```python
from build123d import *

# Parameters (mm, degrees)
BOSS_EXTRUDE1_DEPTH  = 10
FILLET1_R            = 5
SKETCH6_R            = 4.65
BOSS_EXTRUDE2_DEPTH  = 5
SKETCH7_R            = 5
BOSS_EXTRUDE3_DEPTH  = 2
FILLET2_R            = 1
FILLET2_OF_MIRROR1_R = 1
BOSS_EXTRUDE4_START  = -10
BOSS_EXTRUDE4_DEPTH  = 10
SKETCH9_R            = 4.175
CUT_EXTRUDE1_DEPTH   = 5
SKETCH10_R           = 1.175
CUT_EXTRUDE2_DEPTH   = 71.738227722
SKETCH12_W           = 1
SKETCH12_H           = 12
CUT_EXTRUDE3_DEPTH   = 7
CUT_EXTRUDE3_DRAFT   = -2
SKETCH13_W           = 1
SKETCH13_H           = 12
CUT_EXTRUDE4_DEPTH   = 7
CUT_EXTRUDE4_DRAFT   = -2


with BuildPart() as part:
    # Sketch3 → Boss-Extrude1 (new body)
    with BuildSketch(Plane(origin=(0, 0, 0), x_dir=(0, 0, -1), z_dir=(1, 0, 0))):
        with BuildLine():
            Line((-37, -7), (-37, 12.5))
            ThreePointArc((-37, 12.5), (-27.627416998, 35.127416998), (-5, 44.5))
            Line((-5, 44.5), (5, 44.5))
            ThreePointArc((5, 44.5), (27.627416998, 35.127416998), (37, 12.5))
            Line((37, 12.5), (37, -7))
            Line((37, -7), (40, -7))
            Line((40, -7), (40, 12.5))
            ThreePointArc((40, 12.5), (29.748737342, 37.248737342), (5, 47.5))
            Line((5, 47.5), (-5, 47.5))
            ThreePointArc((-5, 47.5), (-29.748737342, 37.248737342), (-40, 12.5))
            Line((-40, 12.5), (-40, -7))
            Line((-40, -7), (-37, -7))
        make_face()
    extrude(amount=BOSS_EXTRUDE1_DEPTH)

    # Fillet1
    fillet1_edges = [part.edges().sort_by_distance(p)[0] for p in [
        (10, -7, -38.5),
        (0, -7, -38.5),
        (0, -7, 38.5),
        (10, -7, 38.5),
    ]]
    fillet(fillet1_edges, radius=FILLET1_R - 0.0001)  # a hair under: the kernel refuses the full size

    # Sketch6 → Boss-Extrude2 (add)
    with BuildSketch(Plane(origin=(0, 0, 37), x_dir=(-1, 0, 0), z_dir=(0, 0, -1))):
        with Locations(Location((-5, 0, 0), (0, 0, 270))):
            Circle(SKETCH6_R)
    boss_extrude2 = extrude(amount=BOSS_EXTRUDE2_DEPTH)

    # Sketch7 → Boss-Extrude3 (add)
    with BuildSketch(Plane(origin=(0, 0, 32), x_dir=(-1, 0, 0), z_dir=(0, 0, -1))):
        with Locations(Location((-5, 0, 0), (0, 0, 90))):
            Circle(SKETCH7_R)
    boss_extrude3 = extrude(amount=BOSS_EXTRUDE3_DEPTH)

    # Fillet2
    fillet2_edges = [part.edges().sort_by_distance(p)[0] for p in [
        (5, -5, 30),
    ]]
    fillet(fillet2_edges, radius=FILLET2_R)

    # Mirror1: Boss-Extrude2, Boss-Extrude3 across plane
    add(boss_extrude2.mirror(Plane.XY))
    add(boss_extrude3.mirror(Plane.XY))

    # Fillet2 of Mirror1
    fillet2_of_mirror1_edges = [part.edges().sort_by_distance(p)[0] for p in [
        (5, -5, -30),
    ]]
    fillet(fillet2_of_mirror1_edges, radius=FILLET2_OF_MIRROR1_R)

    # Sketch8 → Boss-Extrude4 (add)
    with BuildSketch(Plane(origin=(10, 0, 0), x_dir=(0, 0, -1), z_dir=(1, 0, 0)).offset(BOSS_EXTRUDE4_START)):
        with BuildLine():
            Line((8.815238473, 55.479534195), (-8.815238473, 55.479534195))
            add(Edge.make_bspline(
                [(-16.460806571, 45.570378177), (-9.68931269, 49.59059719), (-8.815238473, 55.479534195)],
                knots=[0, 0, 0, 1, 1, 1], degree=2))
            ThreePointArc((-16.460806571, 45.570378177), (-10.811056867, 47.014223417), (-5, 47.5))
            Line((-5, 47.5), (5, 47.5))
            ThreePointArc((5, 47.5), (10.811056867, 47.014223417), (16.460806571, 45.570378177))
            add(Edge.make_bspline(
                [(16.460806571, 45.570378177), (9.68931269, 49.59059719), (8.815238473, 55.479534195)],
                knots=[0, 0, 0, 1, 1, 1], degree=2))
        make_face()
    extrude(amount=BOSS_EXTRUDE4_DEPTH)

    # Sketch9 → Cut-Extrude1 (cut)
    with BuildSketch(Plane(origin=(0, 55.479534195, 0), x_dir=(1, 0, 0), z_dir=(0, 1, 0))):
        with Locations(Location((5, 0, 0), (0, 0, 270))):
            Circle(SKETCH9_R)
    extrude(amount=-CUT_EXTRUDE1_DEPTH, mode=Mode.SUBTRACT)

    # Sketch10 → Cut-Extrude2 (cut, through all)
    with BuildSketch(Plane(origin=(0, 50.479534195, 0), x_dir=(1, 0, 0), z_dir=(0, 1, 0))):
        with Locations(Location((5, 0, 0), (0, 0, 270))):
            Circle(SKETCH10_R)
    extrude(amount=-CUT_EXTRUDE2_DEPTH, mode=Mode.SUBTRACT)


with BuildPart() as cut_extrude3_tool:
    # Sketch12 → Cut-Extrude3 (with draft: the straight prism first)
    with BuildSketch(Plane(origin=(0, 0, 30), x_dir=(-1, 0, 0), z_dir=(0, 0, -1))):
        with Locations((-5, 0)):
            Rectangle(SKETCH12_W, SKETCH12_H)
    extrude(amount=-CUT_EXTRUDE3_DEPTH)
    # Cut-Extrude3: the draft: its side faces are tilted about the plane it starts from
    cut_extrude3_sides = [cut_extrude3_tool.faces().sort_by_distance(p)[0] for p in [
        (4.5, 0, 33.5),
        (5, 6, 33.5),
        (5.5, 0, 33.5),
        (5, -6, 33.5),
    ]]
    draft(cut_extrude3_sides, Plane(origin=(0, 0, 30), x_dir=(-1, 0, 0), z_dir=(0, 0, -1)), CUT_EXTRUDE3_DRAFT)


with BuildPart() as part_1:
    add(part.part)

    # Cut-Extrude3: cut by cut_extrude3_tool
    add(cut_extrude3_tool.part, mode=Mode.SUBTRACT)


with BuildPart() as cut_extrude4_tool:
    # Sketch13 → Cut-Extrude4 (with draft: the straight prism first)
    with BuildSketch(Plane.XY.offset(-30)):
        with Locations((5, 0)):
            Rectangle(SKETCH13_W, SKETCH13_H)
    extrude(amount=-CUT_EXTRUDE4_DEPTH)
    # Cut-Extrude4: the draft: its side faces are tilted about the plane it starts from
    cut_extrude4_sides = [cut_extrude4_tool.faces().sort_by_distance(p)[0] for p in [
        (5, -6, -33.5),
        (5.5, 0, -33.5),
        (5, 6, -33.5),
        (4.5, 0, -33.5),
    ]]
    draft(cut_extrude4_sides, Plane.XY.offset(-30), CUT_EXTRUDE4_DRAFT)


with BuildPart() as part_2:
    add(part_1.part)

    # Cut-Extrude4: cut by cut_extrude4_tool
    add(cut_extrude4_tool.part, mode=Mode.SUBTRACT)


solid = part_2.part
```
CAD build for the part. Positions are in the model's coordinates, mm. A direction names the side the tool comes from. Give positions to 0.01 mm unless a question says otherwise; leave off trailing zeros. Order: outer loops, then holes, each group sorted by start corner. A loop starts at its lowest first (then second) coordinate and runs counter-clockwise, first axis right, second up.
(1) Drill centre lines: L1, parallel to X at y = 48.05, z = 0 (3 decimals); L2, parallel to Z at x = 7, y = 10; L3, parallel to Z at x = 6.75, y = -1. Where is each one in solid material? Low to high.
(2) Saw through at D-D, the plane y = 13.5. Give the cut face in (x, z).
(3) Saw through at B-B, the plane y = 33. Give the cut face in (x, z).
(4) Tool access for faces 1 (the cylindrical face through (0.924, 53.015, -0.905)), 2 (the flat face through (7, 0, -30)), 3 (the cylindrical face through (0.35, -0.1, -34.53)), 4 (the flat face through (9.8, 0, -32)): list every direction of +Z, -Z, +X, -X, +Y, -Y with a clear straight run to the whole face (end or side of a thin tool).
(5) Flat gauge pins, fed straight in: pin 1 (6 mm diameter, centred on x = 8.5, z = -23.5, fed in from -Y); pin 2 (4 mm diameter, centred on x = 7, z = 28.5, fed in from -Y); pin 3 (1.5 mm diameter, centred on x = 6.5, z = 20.5, fed in from +Y). Where does each tip first touch, or does it go through?
(6) Saw through at C-C, the plane z = -34. Give the cut face in (x, y), then the cut area to 3 significant figures.
(7) Saw through at A-A, the plane z = 0. Give the cut face in (x, y) (3 decimals), then the cut area to 3 significant figures.
(8) Mould opens along Y. For faces 5 (the cylindrical face through (0, -0.1, 31.5)), 6 (the flat face through (10, 46, 0)), 7 (the cylindrical face through (4.93, 33.04, 33.34)) say: released by +Y, released by -Y, zero draft, split by the parting line, or undercut.
Results found:
1. L1: x = 0 to 3.825, 6.175 to 10
1. L2: z = -40 to -37, 37 to 40
1. L3: z = -40 to -30, 30 to 40
2. outline: (0, -39.99) - (10, -39.99) - (10, -36.98) - (0, -36.98) - close; (0, 36.98) - (10, 36.98) - (10, 39.99) - (0, 39.99) - close
3. outline: (0, -33.37) - (10, -33.37) - (10, -29.57) - (0, -29.57) - close; (0, 29.57) - (10, 29.57) - (10, 33.37) - (0, 33.37) - close
4. face 1: +Y
4. face 2: +X, -X, -Y
4. face 3: -X
4. face 4: +X
5. pin 1: stops at y = 36.2
5. pin 2: stops at y = -4.6
5. pin 3: stops at y = 44.24
6. outline: (0, 26.03) - (10, 26.03) - (10, 32.1) - (0, 32.1) - close; (4.64, -4.64) - (4.64, 4.64) arc R4.65 ccw to start; (5.36, -4.64) arc R4.65 ccw to (5.36, 4.64) - close
6. area: 122 mm2
7. outline: (0, 44.5) - (3.825, 44.5) - (3.825, 50.48) - (0.825, 50.48) - (0.825, 55.48) - (0, 55.48) - close; (6.175, 44.5) - (10, 44.5) - (10, 55.48) - (9.175, 55.48) - (9.175, 50.48) - (6.175, 50.48) - close
7. area: 54.0 mm2
8. face 5: undercut
8. face 6: zero draft
8. face 7: released by +Y
